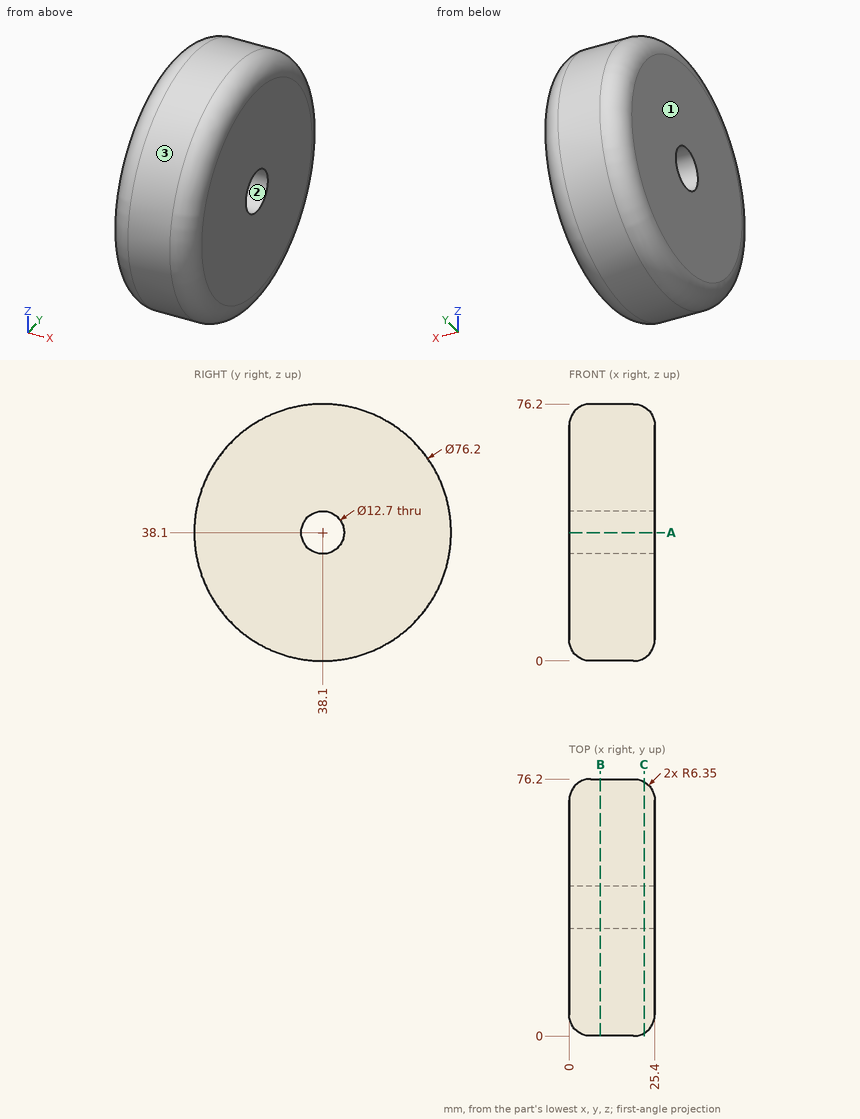
Study the drawing (mm; zero at the part's minimum x, y, z) and answer. Coordinates: 2 decimals unless noted, no trailing zeros. Write each loop counter-clockwise with the first axis right and the second up, starting at its lowest first coordinate (ties: lowest second). Pieces come first, ordered by that corner, then holes. Notation, with made-up numbers: (-13.75, 7) - (12.25, 7) arc R22 ccw to (12.25, 15) - close; hole circle Ø11 at (-10.75, -31.75). An arc over 180 degrees is marked (long way). Put each result on its own line as item: value.
1. Determine the mould class of the marked faces 1, 2 and 3 for opening direction Z: pulls with the +Z half, pulls with the -Z half, needs draft (parallel to the pull), parting line crosses it, or undercut.
Answer sheet:
face 1: needs draft
face 2: undercut
face 3: parting line crosses it
2. The part is cut by section B-B on x = 9.25. Give the vertices of the cut face in (y, z).
Answer sheet:
outline: circle Ø76.2 at (38.1, 38.1); hole circle Ø12.7 at (38.1, 38.1)
3. Find the intervals of material crossed by line 1 along Z through (x, y) = (14.5, 38.1); line 2 along Y through (x, z) = (18, 37); line 3 along Z through (x, y) = (1.5, 32.5), in increasing order. Write a range as from..to.
Answer sheet:
line 1: z = 0..31.75, 44.45..76.2
line 2: y = 0.02..31.85, 44.35..76.18
line 3: z = 2.69..35.11, 41.09..73.51
4. The part is cut by section A-A on z = 38.1. Give the vertices of the cut face in (x, y), plus the area to 3 significant figures.
Answer sheet:
outline: (0, 6.35) arc R6.35 ccw to (6.35, 0) - (19.05, 0) arc R6.35 ccw to (25.4, 6.35) - (25.4, 31.75) - (0, 31.75) - close; (0, 44.45) - (25.4, 44.45) - (25.4, 69.85) arc R6.35 ccw to (19.05, 76.2) - (6.35, 76.2) arc R6.35 ccw to (0, 69.85) - close
area: 1,580 mm^2
5. Flat-ended cylindrical pins translate along their axes: pin 1 Ø2 at (x, y) = (13, 40.5) entering from -Z; pin 2 Ø1 at (x, y) = (6.5, 52) entering from +Z; pin 3 Ø6 at (x, z) = (11.5, 9) entering from +Y. Find the tip coordinate at first contact, or state that the pin passes through.
Answer sheet:
pin 1: stops at z = 0.03
pin 2: stops at z = 73.77
pin 3: stops at y = 65.86
6. The part is cut by section C-C on x = 22.25. Give the vertices of the cut face in (y, z).
Answer sheet:
outline: circle Ø74.47 at (38.1, 38.1); hole circle Ø12.7 at (38.1, 38.1)
